Can you work these out from the model? Positions are in its coordinate system, mm. A direction names the side the tool comes from. Coordinates: 2 decimals unless noted, no trailing zeros. Loops run counter-clockwise (first coordinate to the right, second up) from the corner with the lowest first, then second, coordinate; pieces in that order, holes last. Notation, with made-up numbers: M 69,37.5 L 105,37.5 A19 cw 105,60.5 Z; hole C -28,-6 d1. An arc over 180 degrees is marked long. Answer as a JSON object with one key per item and string values. Group by question number.
Item 1: Suppose I cut it at A-A (y = 42.5). Write out the boundary of the cut face in (x, z), then the cut area to 3 significant figures.
Item 2: Suppose I cut it at D-D (z = -1.5). Write out the boundary of the cut face in (x, y).
Item 3: Suppose I cut it at C-C (x = 13). Write out the boundary of the cut face in (y, z), then the cut area to 3 significant figures.
Item 4: We'd pull the mould along Y, two halves only. Please class faces 1 (the flat face through (-2.5, 26, 12.2)), 2 (the flat face through (0, 26, 18)), 3 (the flat face through (0, 13, -15)): +Y half, -Y half, draft (parallel to the pull), parting line (faces both ways), or undercut.
Item 5: If I drill on line 1 (X direction, y = 19, z = 1); line 2 (Z direction, x = 16, y = 26.5); line 3 (Y direction, x = -29.5, z = 10), over which ranges is the centre line in solid material (lowest first)?
Item 6: I'm going to push flat-ended pins straight in: pin 1 Ø3 at (x, z) = (-3, -11) entering from +Y; pin 2 Ø8 at (x, z) = (-22, 11.5) entering from +Y. Where does each tip first touch, or does it pass through?
Item 7: Which directions (+Z, -Z, +X, -X, +Y, -Y) give clear straight access to the entire face, cutting with the end or side of a thin tool? Please do faces 4 (the flat face through (0, 13, 15)), 5 (the flat face through (-35, 26, 0)), 6 (the flat face through (29, 24, 0)).
Item 8: Suppose I cut it at B-B (z = -13). Write out the boundary of the cut face in (x, y).
Autodesk Inventor part; units mm, degrees
ref_plane "YZ Plane" through (0, 0, 0) normal (1, 0, 0) x (0, 1, 0)
ref_plane "XZ Plane" through (0, 0, 0) normal (0, 1, 0) x (-1, 0, 0)
ref_plane "XY Plane" through (0, 0, 0) normal (0, 0, 1) x (1, 0, 0)
sketch "Boceto1" plane through (0, 0, 0) normal (0, 1, 0) x (-1, 0, 0)
  line L0 (-35, 18) -> (35, 18)
  line L1 (35, 18) -> (35, -18)
  line L2 (35, -18) -> (-35, -18)
  line L3 (-35, -18) -> (-35, 18)
  line L4 (-35, 18) -> (35, -18) construction
  line L5 (35, 18) -> (-35, -18) construction
  line L6 (-32, 15) -> (32, 15)
  line L7 (32, 15) -> (32, -15)
  line L8 (32, -15) -> (-32, -15)
  line L9 (-32, -15) -> (-32, 15)
  line L10 (-32, 15) -> (32, -15) construction
  line L11 (32, 15) -> (-32, -15) construction
  point P0 (0, 0)
  dimension "d0" = 70
  dimension "d1" = 36
  dimension "d2" = 3
  dimension "d3" = 3
extrude "Extrusión1" add sketch "Boceto1" along normal blind 3 contours L6 L7 L8 L9
extrude "Extrusión2" add sketch "Boceto1" along normal blind 23
sketch "Boceto2" plane through (0, 23, 0) normal (0, 1, 0) x (1, 0, 0)
  line L0 (35, 18) -> (-35, 18)
  line L1 (35, -18) -> (-35, -18)
  line L2 (-35, -18) -> (-35, 18)
  line L3 (-35, 18) -> (35, 18)
  line L4 (35, 18) -> (35, -18)
  line L5 (35, -18) -> (-35, 18) construction
  line L6 (-35, -18) -> (35, 18) construction
  line L7 (29, -12) -> (-29, -12)
  line L8 (-29, -12) -> (-29, 12)
  line L9 (-29, 12) -> (29, 12)
  line L10 (29, 12) -> (29, -12)
  line L11 (29, -12) -> (-29, 12) construction
  line L12 (-29, -12) -> (29, 12) construction
  point P0 (0, 0)
  dimension "d8" = 6
  dimension "d9" = 6
extrude "Extrusión3" add sketch "Boceto2" along normal blind 3
sketch "Boceto3" plane through (0, 26, 0) normal (0, 1, 0) x (1, 0, 0)
  point P0 (0, 0)
sketch "Boceto4" plane through (0, 26, 0) normal (0, 1, 0) x (1, 0, 0)
  line L0 (-35, 18) -> (-35, -18)
  line L1 (35, -18) -> (-35, -18)
  line L2 (-35, -18) -> (-35, 18)
  line L3 (-35, 18) -> (35, 18)
  line L4 (35, 18) -> (35, -18)
  line L5 (35, -18) -> (-35, 18) construction
  line L6 (-35, -18) -> (35, 18) construction
  line L7 (32, -15) -> (-32, -15)
  line L8 (-32, -15) -> (-32, 15)
  line L9 (-32, 15) -> (32, 15)
  line L10 (32, 15) -> (32, -15)
  line L11 (32, -15) -> (-32, 15) construction
  line L12 (-32, -15) -> (32, 15) construction
  point P0 (0, 0)
  dimension "d21" = 3
  dimension "d22" = 3
extrude "Extrusión4" add sketch "Boceto4" along normal blind 26
properties part number "Capsula" material "Plástico PET"
From the geometry:
{
 "1": {"outline": "M -35,-18 L 35,-18 L 35,18 L -35,18 Z; hole M -32,-15 L 32,-15 L 32,15 L -32,15 Z", "area": "600 mm2"},
 "2": {"outline": "M -35,0 L 35,0 L 35,52 L 32,52 L 32,26 L 29,26 L 29,23 L 32,23 L 32,3 L -32,3 L -32,23 L -29,23 L -29,26 L -32,26 L -32,52 L -35,52 Z"},
 "3": {"outline": "M 0,-18 L 52,-18 L 52,-15 L 26,-15 L 26,-12 L 23,-12 L 23,-15 L 3,-15 L 3,15 L 23,15 L 23,12 L 26,12 L 26,15 L 52,15 L 52,18 L 0,18 Z", "area": "420 mm2"},
 "4": {"face 1": "+Y half", "face 2": "draft", "face 3": "undercut"},
 "5": {"line 1": "-35 to -32, 32 to 35", "line 2": "-18 to -15, 15 to 18", "line 3": "0 to 3, 23 to 26"},
 "6": {"pin 1": "y = 26", "pin 2": "y = 52"},
 "7": {"face 4": "none", "face 5": "+Z, -Z, -X, +Y, -Y", "face 6": "+Y"},
 "8": {"outline": "M -35,0 L 35,0 L 35,52 L 32,52 L 32,26 L -32,26 L -32,52 L -35,52 Z; hole M -32,3 L 32,3 L 32,23 L -32,23 Z"}
}
